Model file for the job. Use its own axes, mm. Face numbers are marked on the shaded views. A direction names the side the tool comes from. Round coordinates to 2 decimals unless told otherwise and drop trailing zeros. Loops run counter-clockwise (first coordinate to the right, second up) from the corner with the lowest first, then second, coordinate; pieces in that order, holes last. Notation, with made-up numbers: M 43.5,-6.75 L 96.5,-6.75 A26 cw 96.5,22.25 Z; hole C -24,28 d9. An arc over 180 degrees is marked long. Use a Markdown table: item, result. Add a question column.
Item 1: Saw through at B-B on x = 3. Write the cut outline in (y, z), then the cut area to 3 significant figures.
Item 2: Two-plate mould, pull along X, no slides. Class the marked faces 1, 2, 3 and 4: +X half, -X half, draft (parallel to the pull), parting line (faces both ways), or undercut.
Item 3: Pin check, flat tips, straight feed: P1, Ø1.8, axis at x = 7, z = -2, coming from the +Y side; P2, Ø1, axis at x = 3.5, z = -1, coming from the -Y side. Stop position of each tip, or through.
Item 4: Wall check: L1, parallel to Z at x = 1.25, y = 1.75; L2, parallel to Y at x = 7, z = -2; L3, parallel to Y at x = 13, z = -2.75. Give the ranges that are in metal, low to high. Write a range as from..to.
Item 5: Tool access for the marked faces 5 and 6: list every direction of +Z, -Z, +X, -X, +Y, -Y with a clear straight run to the whole face (end or side of a thin tool).
Item 6: Saw through at D-D on z = -5. Write the cut outline in (x, y).
Item 7: Saw through at C-C on x = 8.25. Write the cut outline in (y, z).
Item 8: Saw through at A-A on z = -1.75. Write the cut outline in (x, y).
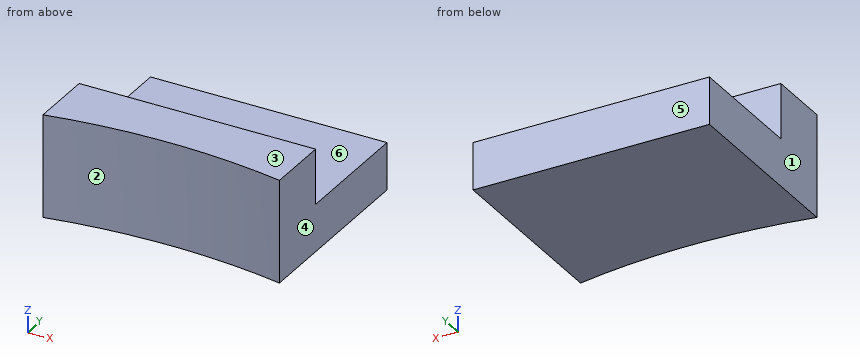
```python
from build123d import *

# Parameters (mm, degrees)
SKETCH1_W           = 15
SKETCH1_H           = 6.5
BOSS_EXTRUDE1_DEPTH = 1
BOSS_EXTRUDE2_START = -6.5
BOSS_EXTRUDE2_DEPTH = 6.5
SKETCH3_W           = 15
SKETCH3_H           = 3
BOSS_EXTRUDE3_DEPTH = 8


with BuildPart() as part:
    # Sketch1 → Boss-Extrude1 (new body)
    with BuildSketch(Plane(origin=(0, 0, 0), x_dir=(1, 0, 0), z_dir=(0, 1, 0))):
        with Locations((7.5, 3.25)):
            Rectangle(SKETCH1_W, SKETCH1_H)
    extrude(amount=BOSS_EXTRUDE1_DEPTH)

    # Sketch2 → Boss-Extrude2 (add)
    with BuildSketch(Plane.XY.offset(BOSS_EXTRUDE2_START)):
        with BuildLine():
            Line((0, 0), (0, -3.050294479))
            ThreePointArc((0, -3.050294479), (7.5, -2.340878593), (15, -3.050294479))
            Line((15, -3.050294479), (15, 0))
            ThreePointArc((15, 0), (7.5, 0.659121407), (0, 0))
        make_face()
    extrude(amount=BOSS_EXTRUDE2_DEPTH)

    # Sketch3 → Boss-Extrude3 (add)
    with BuildSketch(Plane(origin=(0, 1, 0), x_dir=(1, 0, 0), z_dir=(0, 1, 0))):
        with Locations((7.5, 5)):
            Rectangle(SKETCH3_W, SKETCH3_H)
    extrude(amount=BOSS_EXTRUDE3_DEPTH)


solid = part.part
```
Entries:
| question | item | result |
|---|---|---|
| 1 | outline | M -2.59,-6.5 L 9,-6.5 L 9,-3.5 L 1,-3.5 L 1,0 L -2.59,0 Z |
| 1 | area | 47.4 mm2 |
| 2 | face 1 | -X half |
| 2 | face 2 | undercut |
| 2 | face 3 | draft |
| 2 | face 4 | +X half |
| 3 | P1 | y = 1 |
| 3 | P2 | y = -2.59 |
| 4 | L1 | -6.5..-3.5 |
| 4 | L2 | -2.34..1 |
| 4 | L3 | -2.72..1 |
| 5 | face 5 | +Z, -Z, +X, -X, +Y |
| 5 | face 6 | +Z, +X, -X, +Y |
| 6 | outline | M 0,-3.05 A40 cw 15,-3.05 L 15,9 L 0,9 Z |
| 7 | outline | M -2.35,-6.5 L 9,-6.5 L 9,-3.5 L 1,-3.5 L 1,0 L -2.35,0 Z |
| 8 | outline | M 0,-3.05 A40 cw 15,-3.05 L 15,1 L 0,1 Z |
